from build123d import *

# Parameters (mm, degrees)
F0_W     = 30.48
F0_H     = 30.48
F1_DEPTH = 25.4
F2_DEPTH = 1.27
F3_SIZE  = 12.7
F4_SIZE  = 12.7


with BuildPart() as f1:
    # F0 (on Front) → F1 (new body)
    with BuildSketch(Plane.XZ):
        Polygon((57.15, 82.55), (57.15, 101.6), (38.1, 101.6), (-38.1, 101.6), (-57.15, 101.6), (-57.15, 82.55), (-57.15, 0), (-57.15, -82.55), (-57.15, -101.6), (-38.1, -101.6), (38.1, -101.6), (57.15, -101.6), (57.15, -82.55), (57.15, 0), align=None)
        with Locations((-22.86, -67.31)):
            Rectangle(F0_W, F0_H, mode=Mode.SUBTRACT)
        Polygon((-38.1, -15.24), (-38.1, 0), (-38.1, 15.24), (-7.62, 15.24), (-7.62, -15.24), align=None, mode=Mode.SUBTRACT)
        with Locations((22.86, -67.31)):
            Rectangle(F0_W, F0_H, mode=Mode.SUBTRACT)
        Polygon((38.1, 15.24), (38.1, 0), (38.1, -15.24), (7.62, -15.24), (7.62, 15.24), align=None, mode=Mode.SUBTRACT)
        with Locations((-22.86, 67.31)):
            Rectangle(F0_W, F0_H, mode=Mode.SUBTRACT)
        with Locations((22.86, 67.31)):
            Rectangle(F0_W, F0_H, mode=Mode.SUBTRACT)
    extrude(amount=F1_DEPTH)

    # F0 (on Front) → F2 (join)
    with BuildSketch(Plane.XZ):
        with Locations((-22.86, 67.31)):
            Rectangle(F0_W, F0_H)
        with Locations((22.86, 67.31)):
            Rectangle(F0_W, F0_H)
        Polygon((-38.1, 15.24), (-38.1, 0), (-38.1, -15.24), (-7.62, -15.24), (-7.62, 15.24), align=None)
        Polygon((38.1, -15.24), (38.1, 0), (38.1, 15.24), (7.62, 15.24), (7.62, -15.24), align=None)
        with Locations((-22.86, -67.31)):
            Rectangle(F0_W, F0_H)
        with Locations((22.86, -67.31)):
            Rectangle(F0_W, F0_H)
    extrude(amount=F2_DEPTH)

    # F3
    f3_edges = [f1.edges().sort_by_distance(p)[0] for p in [
        (0, 0, -101.6),
    ]]
    chamfer(f3_edges, length=F3_SIZE)

    # F4
    f4_edges = [f1.edges().sort_by_distance(p)[0] for p in [
        (-57.15, 0, 6.35),
        (0, 0, 101.6),
        (57.15, 0, 6.35),
    ]]
    chamfer(f4_edges, length=F4_SIZE)


solid = f1.part
Here's how the part is built. I have some questions about the finished solid (model axes, mm). A direction names the side the tool comes from. Round coordinates to 2 decimals unless told otherwise and drop trailing zeros. Order: outer loops, then holes, each group sorted by start corner. A loop starts at its lowest first (then second) coordinate and runs counter-clockwise, first axis right, second up. Notation, with made-up numbers: M 52,80.5 L 86,80.5 A19 cw 86,92.5 Z; hole C -4.75,87 d2. An arc over 180 degrees is marked long. Return JSON: item names as keys, results as strings. Group by question number.
1. If we section it at B-B on x = 15: List the corners of the cut face in (y, z) for me, then the cut area to 3 significant figures.
2. If we section it at D-D on y = -9.75: List the corners of the cut face in (x, z) for me, then the cut area to 3 significant figures.
3. If we section it at A-A on y = -21.5: List the corners of the cut face in (x, z) for me.
4. If we mould it in two halves opening along X, with no side actions, what happens to faces 1 (the face through (23, -13, 52.07)), 2 (the face through (-1, -19, -101.6)), 3 (the face through (57.15, -19, -1)), 4 (the face through (-23, -13, -82.55))? For each: pulls with the +X half, pulls with the -X half, needs draft (parallel to the pull), parting line crosses it, or undercut.
5. Please list where these lines run through material, in increasing order: probe 1 along Z at (x, y) = (28.5, -14.25); probe 2 along X at (y, z) = (-17.5, 67); probe 3 along X at (y, z) = (-11.75, -63).
6. If we section it at C-C on z = -65.5: List the corners of the cut face in (x, y) for me.
7. On a 3-axis mill with a long thin cutter (end or side, diameter ignored), from which of +Z, -Z, +X, -X, +Y, -Y can I reach the whole of each face in a straight line? I mean faces 5 (the face through (0.8, -6.4, 95.3)), 6 (the face through (38.1, -13, 0)). Say none if no direction works.
8. I'm going to push flat-ended pins straight in: pin 1 Ø7 at (y, z) = (-8, -60) entering from -X; pin 2 Ø15 at (x, z) = (-26.5, 64) entering from -Y; pin 3 Ø2 at (y, z) = (-11.5, -75) entering from -X. Where does each tip first touch, or does it pass through?
Reply:
{
 "1": {"outline": "M -25.4,-101.6 L -12.7,-101.6 L 0,-88.9 L 0,88.9 L -12.7,101.6 L -25.4,101.6 L -25.4,82.55 L -1.27,82.55 L -1.27,52.07 L -25.4,52.07 L -25.4,15.24 L -1.27,15.24 L -1.27,-15.24 L -25.4,-15.24 L -25.4,-52.07 L -1.27,-52.07 L -1.27,-82.55 L -25.4,-82.55 Z", "area": "2,790 mm^2"},
 "2": {"outline": "M -54.2,-98.65 L 54.2,-98.65 L 54.2,98.65 L -54.2,98.65 Z; hole M -38.1,-82.55 L -7.62,-82.55 L -7.62,-52.07 L -38.1,-52.07 Z; hole M -38.1,-15.24 L -7.62,-15.24 L -7.62,15.24 L -38.1,15.24 Z; hole M -38.1,52.07 L -7.62,52.07 L -7.62,82.55 L -38.1,82.55 Z; hole M 7.62,-82.55 L 38.1,-82.55 L 38.1,-52.07 L 7.62,-52.07 Z; hole M 7.62,-15.24 L 38.1,-15.24 L 38.1,15.24 L 7.62,15.24 Z; hole M 7.62,52.07 L 38.1,52.07 L 38.1,82.55 L 7.62,82.55 Z", "area": "15,800 mm^2"},
 "3": {"outline": "M -57.15,-101.6 L 57.15,-101.6 L 57.15,101.6 L -57.15,101.6 Z; hole M -38.1,-82.55 L -7.62,-82.55 L -7.62,-52.07 L -38.1,-52.07 Z; hole M -38.1,-15.24 L -7.62,-15.24 L -7.62,15.24 L -38.1,15.24 Z; hole M -38.1,52.07 L -7.62,52.07 L -7.62,82.55 L -38.1,82.55 Z; hole M 7.62,-82.55 L 38.1,-82.55 L 38.1,-52.07 L 7.62,-52.07 Z; hole M 7.62,-15.24 L 38.1,-15.24 L 38.1,15.24 L 7.62,15.24 Z; hole M 7.62,52.07 L 38.1,52.07 L 38.1,82.55 L 7.62,82.55 Z"},
 "4": {"face 1": "undercut", "face 2": "needs draft", "face 3": "pulls with the +X half", "face 4": "undercut"},
 "5": {"probe 1": "-101.6 to -82.55, -52.07 to -15.24, 15.24 to 52.07, 82.55 to 101.6", "probe 2": "-57.15 to -38.1, -7.62 to 7.62, 38.1 to 57.15", "probe 3": "-56.2 to -38.1, -7.62 to 7.62, 38.1 to 56.2"},
 "6": {"outline": "M -57.15,-25.4 L -38.1,-25.4 L -38.1,-1.27 L -7.62,-1.27 L -7.62,-25.4 L 7.62,-25.4 L 7.62,-1.27 L 38.1,-1.27 L 38.1,-25.4 L 57.15,-25.4 L 57.15,-12.7 L 44.45,0 L -44.45,0 L -57.15,-12.7 Z"},
 "7": {"face 5": "+Z, +X, -X, +Y", "face 6": "-Y"},
 "8": {"pin 1": "x = -55.95", "pin 2": "y = -1.27", "pin 3": "x = -56.95"}
}
